Verification items for the finished model (mm, model axes). A direction names the side the tool comes from. Coordinates: 2 decimals unless noted, no trailing zeros. Order: outer loops, then holes, each group sorted by start corner. A loop starts at its lowest first (then second) coordinate and runs counter-clockwise, first axis right, second up. Notation, with made-up numbers: M 83,3 L 95,3 A15 ccw 95,18 Z; hole C 28.25,50 d8. An arc over 180 degrees is marked long. Write item = value, one per line.
Autodesk Inventor part; units mm, degrees
ref_plane "YZ Plane" through (0, 0, 0) normal (1, 0, 0) x (0, 1, 0)
ref_plane "XZ Plane" through (0, 0, 0) normal (0, 1, 0) x (-1, 0, 0)
ref_plane "XY Plane" through (0, 0, 0) normal (0, 0, 1) x (1, 0, 0)
sketch "Sketch1" plane through (0, 0, 0) normal (0, 0, 1) x (1, 0, 0)
  line L0 (0, 0) -> (0, 13)
  line L1 (0, 13) -> (24, 13)
  line L2 (24, 13) -> (24, 0)
  line L3 (24, 0) -> (22, 0)
  line L4 (22, 0) -> (22, 10)
  line L5 (22, 10) -> (2, 10)
  line L6 (2, 10) -> (2, 0)
  line L7 (2, 0) -> (0, 0)
  dimension "d0" = 13
  dimension "d1" = 24
  dimension "d2" = 2
  dimension "d3" = 10
  dimension "d4" = 20
revolve "Revolution1" add sketch "Sketch1" angle 360 about axis through (0, 13, 0) along (1, 0, 0)
sketch "Sketch2" plane through (2, 13, 0) normal (1, 0, 0) x (0, 0, -1)
  point P0 (0, -13)
  point P1 (-3.9905, -0.6009)
hole "Hole1" at (2, 12.3991, 3.9905) direction (-1, 0, 0) diameter 2 end through all
sketch "Sketch3" plane through (24, 13, 0) normal (1, 0, 0) x (0, 0, -1)
  point P0 (0, -13)
  point P1 (-10.0295, -1.8525)
hole "Hole2" at (24, 11.1475, 10.0295) direction (-1, 0, 0) diameter 2 depth 8 tip angle 118
sketch "Sketch4" plane through (2, 13, 0) normal (1, 0, 0) x (0, 0, -1)
  point P0 (0, -13)
sketch "Sketch5" plane through (2, 13, 0) normal (1, 0, 0) x (0, 0, -1)
  point P0 (0, -13)
sketch "Sketch6" plane through (0, 13, 0) normal (-1, 0, 0) x (0, 0, 1)
  point P0 (0, -13)
properties part number "SpoolNoCenterHole1"
Item 1: Tool access check on faces 4 (the cylindrical face through (23, 0.6, 3.9)), 5 (the cylindrical face through (0.99, 13.01, 4.78)). Record the directions out of +Z, -Z, +X, -X, +Y, -Y that give a thin tool (end or side, any length) a straight path to the whole face; none if there is none.
Report:
face_4 = +X, -X
face_5 = -X
Item 2: Sectioned sample at D-D, the plane y = 13. Enter the section's corners in (x, z), then the cut area to 3 significant figures.
Report:
outline = M 0,-13 L 2,-13 L 2,-3 L 22,-3 L 22,-13 L 24,-13 L 24,13 L 22,13 L 22,3 L 2,3 L 2,3.19 L 0,3.19 Z; M 0,4.79 L 2,4.79 L 2,13 L 0,13 Z
area = 221 mm^2
Item 3: Sectioned sample at A-A, the plane y = 24. Enter the section's corners in (x, z), then the cut area to 3 significant figures.
Report:
outline = M 0,-6.93 L 2,-6.93 L 2,6.93 L 0,6.93 Z; M 22,-6.93 L 24,-6.93 L 24,6.93 L 22,6.93 Z
area = 55.4 mm^2
Item 4: Scan lines: L1, parallel to X at y = 6.5, z = -5.5; L2, parallel to Z at x = 13, y = 13.75; L3, parallel to Z at x = 21.5, y = 11. Record each from-to range of solid material in increasing order. Write a range as from..to.
Report:
L1 = 0..2, 22..24
L2 = -2.9..2.9
L3 = -2.24..2.24
Item 5: Sectioned sample at C-C, the plane z = 0. Enter the section's corners in (x, y).
Report:
outline = M 0,0 L 2,0 L 2,10 L 22,10 L 22,0 L 24,0 L 24,26 L 22,26 L 22,16 L 2,16 L 2,26 L 0,26 Z
Item 6: Release check for a two-part mould opening along Y. For faces 1 (the flat face through (24, 13, 0)), 2 (the cylindrical face through (12, 16, 0)), 3 (the cylindrical face through (22.986, 12.035, 9.568)) record: pulls with the +Y half, pulls with the -Y half, needs draft (parallel to the pull), parting line crosses it, or undercut.
Report:
face_1 = needs draft
face_2 = parting line crosses it
face_3 = undercut
Item 7: Sectioned sample at B-B, the plane z = -4.5. Enter the section's corners in (x, y).
Report:
outline = M 0,0.8 L 2,0.8 L 2,25.2 L 0,25.2 Z; M 22,0.8 L 24,0.8 L 24,25.2 L 22,25.2 Z
Item 8: Gauge pin test, flat end, axial feed: pin 1 (5 mm diameter, centred on x = 10, z = -2.5, fed in from -Y). Record the tip position at first contact, or that the pin passes through.
Report:
pin_1 = 10
